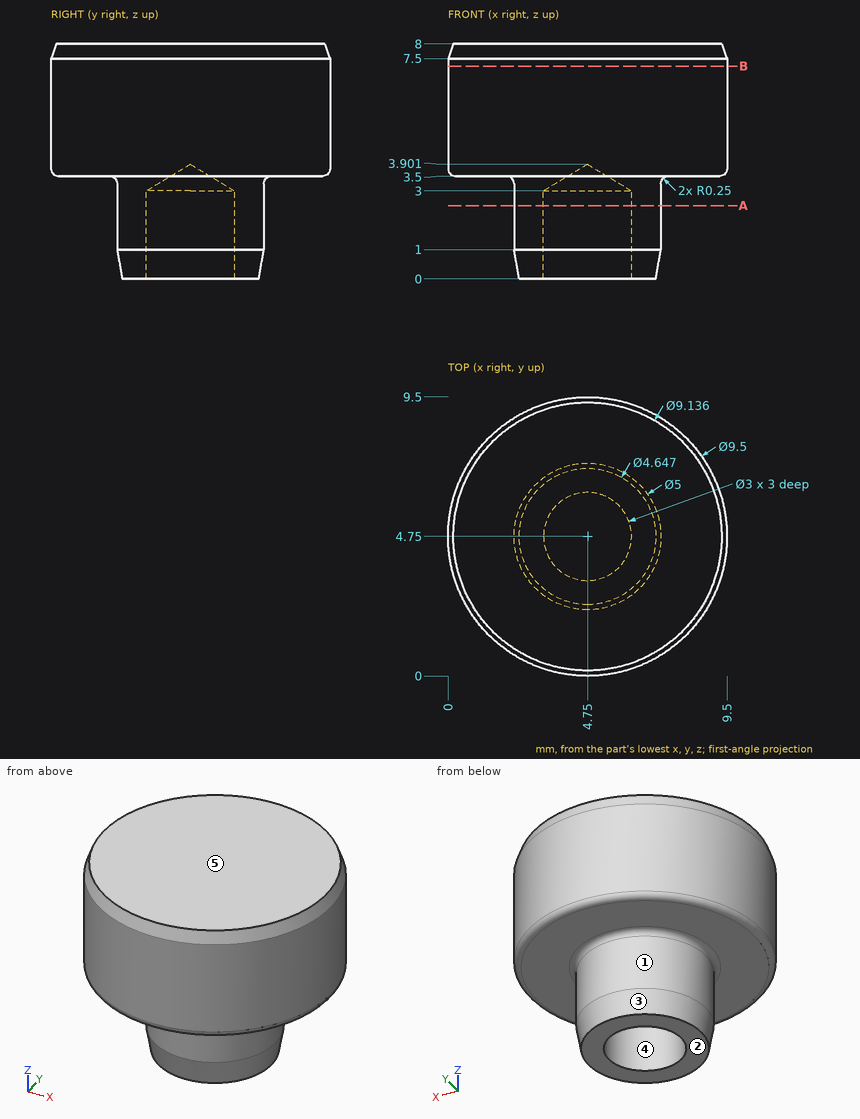
Could you check a few things on this drawing? It's one solid part, dimensions in mm from its lowest x, y, z. A direction names the side the tool comes from. Coordinates: 2 decimals unless noted, no trailing zeros. Order: outer loops, then holes, each group sorted by start corner. A loop starts at its lowest first (then second) coordinate and runs counter-clockwise, first axis right, second up. Notation, with made-up numbers: (-1.75, 7.5) - (35.25, 7.5) arc R9 cw to (35.25, 20.5) - close; hole circle Ø1 at (-15, 26). An arc over 180 degrees is marked (long way). One line per question, with ' | ' between items.
(1) If I drill on L1, parallel to X at y = 4.75, z = 1.6; L2, parallel to Z at x = 6.25, y = 8, over which ranges is the centre line in solid material (lowest first)?
Report:
L1: x = 2.25 to 3.25, 6.25 to 7.25 | L2: z = 3.5 to 8
(2) Suppose I cut it at A-A on z = 2.5. List the corners of the cut face in (x, y) for me.
Report:
outline: circle Ø5 at (4.75, 4.75); hole circle Ø3 at (4.75, 4.75)
(3) Suppose I cut it at B-B on z = 7.25. List the corners of the cut face in (x, y) for me.
Report:
outline: circle Ø9.5 at (4.75, 4.75)
(4) If we mould it in two halves opening along Y, with no side actions, what happens to the marked faces 3, 4 and 5? For each: pulls with the +Y half, pulls with the -Y half, needs draft (parallel to the pull), parting line crosses it, or undercut.
Report:
face 3: parting line crosses it | face 4: undercut | face 5: needs draft
(5) Will these pins go through, and if not, where does the flat tip stop? pin 1 (1.5 mm diameter, centred on y = 6.5, z = 3, fed in from +X) (1 decimal); pin 2 (4 mm diameter, centred on y = 2.5, z = 3.5, fed in from +X); pin 3 (2 mm diameter, centred on x = 3, z = 5, fed in from -Y).
Report:
pin 1: stops at x = 9.3 | pin 2: stops at x = 9.49 | pin 3: stops at y = 0.06
(6) For the marked faces 1 and 2, which set-ups out of +Z, -Z, +X, -X, +Y, -Y let a thin tool reach every point of the face, with its end or its side?
Report:
face 1: -Z | face 2: -Z, +X, -X, +Y, -Y
